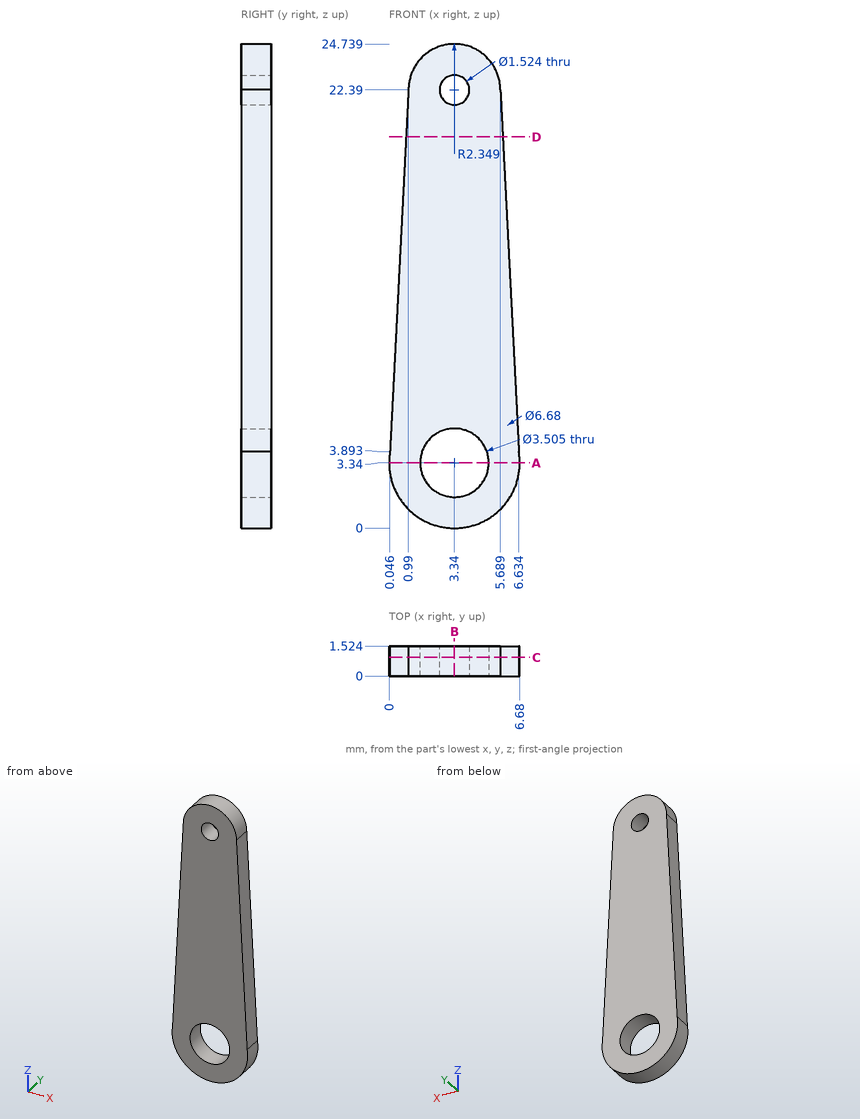
For this review, use the dimensioned drawing (mm, ordinates from the lowest corner) and the shaded views. Give positions to 0.01 mm unless a question says otherwise; leave off trailing zeros. Loops run counter-clockwise (first coordinate to the right, second up) from the corner with the lowest first, then second, coordinate; pieces in that order, holes last.
Item 1: Take a section at C-C, the plane y = 0.95. Give the number of separate pieces and of enclosed holes in the cut face, and give its area (3 significant figures).
Item 2: Take a section at A-A, the plane z = 3.34. State the section outline as (x, y) points (1 decimal).
Item 3: Take a section at D-D, the plane z = 20. State the section outline as (x, y) points (1 decimal).
Item 4: For line 1 along Z through (x, y) = (3.34, 0.8); line 2 along Z through (x, y) = (3.5, 0.65) (1 decimal); line 3 along Z through (x, y) = (4.75, 0.35) (1 decimal), list the stretches that pass through material, from the lowest coordinate up.
Item 5: Take a section at B-B, the plane x = 3.34. State the section outline as (y, z) points (1 decimal).
Item 6: Insertion check: pin 1 (1.4 mm diameter, centred on x = 3.34, z = 22.39, fed in from +Y). The pin has a flat end and moves straight along its axis. Give the tip position at first contact, or say it passes through.
Calculated:
1. separate pieces: 1
1. enclosed holes: 2
1. area: 123 mm2
2. outline: (0, 0) - (1.6, 0) - (1.6, 1.5) - (0, 1.5) - close; (5.1, 0) - (6.7, 0) - (6.7, 1.5) - (5.1, 1.5) - close
3. outline: (0.9, 0) - (5.8, 0) - (5.8, 1.5) - (0.9, 1.5) - close
4. line 1: z = 0 to 1.59, 5.09 to 21.63, 23.15 to 24.74
4. line 2: z = 0 to 1.6, 5.1 to 21.6, 23.1 to 24.7
4. line 3: z = 0.3 to 2.3, 4.4 to 24.3
5. outline: (0, 0) - (1.5, 0) - (1.5, 1.6) - (0, 1.6) - close; (0, 5.1) - (1.5, 5.1) - (1.5, 21.6) - (0, 21.6) - close; (0, 23.2) - (1.5, 23.2) - (1.5, 24.7) - (0, 24.7) - close
6. pin 1: passes through
